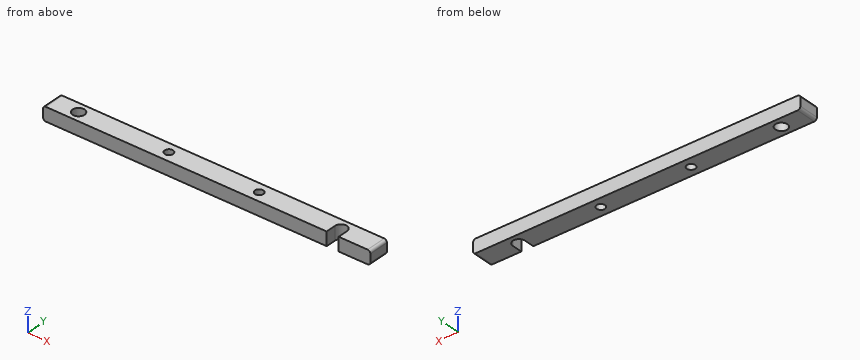
```python
from build123d import *

# Parameters (mm, degrees)
SKETCH1_W               = 304.8
SKETCH1_H               = 19.05
BOSS_EXTRUDE1_DEPTH     = 6.35
CUT_EXTRUDE1_DEPTH      = 154.224592103
CUT_EXTRUDE1_DEPTH_BACK = 154.224592103
SKETCH2_R               = 5.588
SKETCH2_R_2             = 3.937
FILLET1_R               = 2.54


with BuildPart() as part:
    # Sketch1 → Boss-Extrude1 (new, symmetric)
    with BuildSketch(Plane.XY):
        Rectangle(SKETCH1_W, SKETCH1_H)
    extrude(amount=BOSS_EXTRUDE1_DEPTH, both=True)

    # Sketch2 → Cut-Extrude1 (cut, two sides: drawn at the far end of the back side and taken through both)
    with BuildSketch(Plane.XY.offset(6.35).offset(-CUT_EXTRUDE1_DEPTH_BACK)):
        with BuildLine():
            Line((122.936, -9.525), (122.936, 0))
            ThreePointArc((122.936, 0), (117.348, 5.588), (111.76, 0))
            Line((111.76, 0), (111.76, -9.525))
            Line((111.76, -9.525), (122.936, -9.525))
        make_face()
        with Locations((-127, 0)):
            Circle(SKETCH2_R)
        with Locations((-42.926, 0)):
            Circle(SKETCH2_R_2)
        with Locations((41.148, 0)):
            Circle(SKETCH2_R_2)
    extrude(amount=CUT_EXTRUDE1_DEPTH + CUT_EXTRUDE1_DEPTH_BACK, mode=Mode.SUBTRACT)

    # Fillet1
    fillet1_edges = [part.edges().sort_by_distance(p)[0] for p in [
        (-152.4, 0, 6.35),
        (152.4, 0, 6.35),
        (-152.4, 0, -6.35),
        (152.4, 0, -6.35),
    ]]
    fillet(fillet1_edges, radius=FILLET1_R)


solid = part.part
```
Read the model definition and answer for the solid it produces. Units are mm, in the model's axes. Coordinates: 2 decimals unless noted, no trailing zeros. Loops run counter-clockwise (first coordinate to the right, second up) from the corner with the lowest first, then second, coordinate; pieces in that order, holes last.
(1) The part is cut by section C-C (x = -42). Determine the outline of the cut face in (y, z) (3 decimals), and give its area (3 significant figures).
Solution:
outline: (-9.525, -6.35) - (-3.827, -6.35) - (-3.827, 6.35) - (-9.525, 6.35) - close; (3.827, -6.35) - (9.525, -6.35) - (9.525, 6.35) - (3.827, 6.35) - close
area: 145 mm2
(2) Consider line 1 along X through (y, z) = (-1.5, 3); line 2 along X through (y, z) = (-3.25, -1.75); line 3 along X through (y, z) = (-5.75, -0.25). Determine where each line is inside the solid, lowest interval first.
Solution:
line 1: x = -152.4 to -132.38, -121.62 to -46.57, -39.29 to 37.51, 44.79 to 111.76, 122.94 to 152.4
line 2: x = -152.4 to -131.55, -122.45 to -45.15, -40.7 to 38.93, 43.37 to 111.76, 122.94 to 152.4
line 3: x = -152.4 to 111.76, 122.94 to 152.4
(3) The part is cut by section D-D (x = 119.5). Determine the outline of the cut face in (y, z) (3 decimals).
Solution:
outline: (5.157, -6.35) - (9.525, -6.35) - (9.525, 6.35) - (5.157, 6.35) - close
(4) The part is cut by section A-A (x = -127). Determine the outline of the cut face in (y, z) (3 decimals), and give its area (4 significant figures).
Solution:
outline: (-9.525, -6.35) - (-5.588, -6.35) - (-5.588, 6.35) - (-9.525, 6.35) - close; (5.588, -6.35) - (9.525, -6.35) - (9.525, 6.35) - (5.588, 6.35) - close
area: 100.0 mm2
(5) The part is cut by section B-B (z = -1.75). Determine the outline of the cut face in (x, y) (3 decimals), and give its area (3 significant figures).
Solution:
outline: (-152.4, -9.525) - (111.76, -9.525) - (111.76, 0) arc R5.588 cw to (122.936, 0) - (122.936, -9.525) - (152.4, -9.525) - (152.4, 9.525) - (-152.4, 9.525) - close; hole circle Ø11.176 at (-127, 0); hole circle Ø7.874 at (-42.926, 0); hole circle Ø7.874 at (41.148, 0)
area: 5,460 mm2
(6) Flat-ended cylindrical pins translate along their axes: pin 1 Ø7 at (x, y) = (41.148, 0) entering from +Z; pin 2 Ø1.5 at (y, z) = (0.5, 5) entering from -X; pin 3 Ø1 at (y, z) = (-2.5, 4.5) entering from +X. Find the tip coordinate at first contact, or state that the pin passes through.
Solution:
pin 1: passes through
pin 2: stops at x = -152.36
pin 3: stops at x = 152.39
